```python
from build123d import *

# Parameters (mm, degrees)
SKETCH1_W            = 91.5
SKETCH1_H            = 100
BOSS_EXTRUDE1_DEPTH  = 3
M4_CLEARANCE_HOLE1_D = 4.3
M3_CLEARANCE_HOLE1_D = 3.2
SKETCH6_W            = 15
SKETCH6_H            = 35
CUT_EXTRUDE1_DEPTH   = 107.30733747
FILLET1_R            = 3


with BuildPart() as part:
    # Sketch1 → Boss-Extrude1 (new body)
    with BuildSketch(Plane.XY):
        with Locations((10.75, 40)):
            Rectangle(SKETCH1_W, SKETCH1_H)
    extrude(amount=BOSS_EXTRUDE1_DEPTH)

    # M4 Clearance Hole1 (through all)
    with Locations(Plane.XY.offset(3)):
        with Locations((-25, 0), (25, 0)):
            Hole(M4_CLEARANCE_HOLE1_D / 2)

    # M3 Clearance Hole1 (through all)
    with Locations(Plane.XY.offset(3)):
        with Locations((-8.5, 80), (46.5, 80)):
            Hole(M3_CLEARANCE_HOLE1_D / 2)

    # Sketch6 → Cut-Extrude1 (cut, through all)
    with BuildSketch(Plane.XY.offset(3)):
        with Locations((-27.5, 72.5)):
            Rectangle(SKETCH6_W, SKETCH6_H)
    extrude(amount=-CUT_EXTRUDE1_DEPTH, mode=Mode.SUBTRACT)

    # Fillet1
    fillet1_edges = [part.edges().sort_by_distance(p)[0] for p in [
        (-20, 90, 1.5),
        (-20, 55, 1.5),
        (-35, 55, 1.5),
        (56.5, 90, 1.5),
        (56.5, -10, 1.5),
        (-35, -10, 1.5),
    ]]
    fillet(fillet1_edges, radius=FILLET1_R)


solid = part.part
```
The model under review builds one solid part; all positions refer to its coordinate system, in mm. A direction names the side the tool comes from. Round coordinates to 2 decimals unless told otherwise and drop trailing zeros. Order: outer loops, then holes, each group sorted by start corner. A loop starts at its lowest first (then second) coordinate and runs counter-clockwise, first axis right, second up. Notation, with made-up numbers: (-1.75, 4.25) -> (26.25, 4.25) arc R21 cw to (26.25, 33.25) -> close; hole circle Ø5 at (-26, 35). An arc over 180 degrees is marked (long way). Use a Markdown table: item, result.
Q1. We need section D-D on x = 46.5. Write out the cut boundary in (y, z), then the cut area to 3 significant figures.
Values:
| item | result |
|---|---|
| outline | (-10, 0) -> (78.4, 0) -> (78.4, 3) -> (-10, 3) -> close; (81.6, 0) -> (90, 0) -> (90, 3) -> (81.6, 3) -> close |
| area | 290 mm^2 |
Q2. For line 1 (X direction, y = 80, z = 2.35); line 2 (Y direction, x = -8.5, z = 1.45); line 3 (Y direction, x = 25, z = 1.85), list the stretches that pass through material, from the lowest coordinate up.
Values:
| item | result |
|---|---|
| line 1 | x = -20 to -10.1, -6.9 to 44.9, 48.1 to 56.5 |
| line 2 | y = -10 to 78.4, 81.6 to 90 |
| line 3 | y = -10 to -2.15, 2.15 to 90 |
Q3. Mouldability with a two-part tool opening along X and no side actions: class faces 1 (the cylindrical face through (44.974, 80.481, 1.479)), 2 (the cylindrical face through (-34.14, 54.1, 1.48)), 3 (the cylindrical face through (22.95, 0.65, 1.48)), 4 (the cylindrical face through (55.6, 89.14, 1.52)) as +X half, -X half, draft (parallel to the pull), parting line (faces both ways), or undercut.
Values:
| item | result |
|---|---|
| face 1 | undercut |
| face 2 | -X half |
| face 3 | undercut |
| face 4 | +X half |
Q4. Clearance check with flat-ended pins moving along their axes: P1, Ø0.9, axis at x = -29, z = 1, coming from the +Y side; P2, Ø10, axis at x = 23, y = 25, coming from the -Z side. State where each tip first meets the part, or that it passes through.
Values:
| item | result |
|---|---|
| P1 | stops at y = 55 |
| P2 | stops at z = 0 |
Q5. We need section C-C on z = 2.3. Write out the cut boundary in (x, y), then the cut area to 3 significant figures.
Values:
| item | result |
|---|---|
| outline | (-35, -7) arc R3 ccw to (-32, -10) -> (53.5, -10) arc R3 ccw to (56.5, -7) -> (56.5, 87) arc R3 ccw to (53.5, 90) -> (-17, 90) arc R3 ccw to (-20, 87) -> (-20, 58) arc R3 cw to (-23, 55) -> (-32, 55) arc R3 ccw to (-35, 52) -> close; hole circle Ø4.3 at (-25, 0); hole circle Ø3.2 at (-8.5, 80); hole circle Ø4.3 at (25, 0); hole circle Ø3.2 at (46.5, 80) |
| area | 8,570 mm^2 |
Q6. We need section A-A on x = 25. Write out the cut boundary in (y, z), then the cut area to 3 significant figures.
Values:
| item | result |
|---|---|
| outline | (-10, 0) -> (-2.15, 0) -> (-2.15, 3) -> (-10, 3) -> close; (2.15, 0) -> (90, 0) -> (90, 3) -> (2.15, 3) -> close |
| area | 287 mm^2 |
Q7. Tool access review of faces 5 (the flat face through (10, -10, 1)), 6 (the flat face through (-28, 55, 2)): name each direction out of +Z, -Z, +X, -X, +Y, -Y from which nothing blocks a thin tool from reaching the whole face with its end or side.
Values:
| item | result |
|---|---|
| face 5 | +Z, -Z, +X, -X, -Y |
| face 6 | +Z, -Z, -X, +Y |
Q8. We need section B-B on y = 80. Write out the cut boundary in (x, z), then the cut area to 3 significant figures.
Values:
| item | result |
|---|---|
| outline | (-20, 0) -> (-10.1, 0) -> (-10.1, 3) -> (-20, 3) -> close; (-6.9, 0) -> (44.9, 0) -> (44.9, 3) -> (-6.9, 3) -> close; (48.1, 0) -> (56.5, 0) -> (56.5, 3) -> (48.1, 3) -> close |
| area | 210 mm^2 |
